```python
from build123d import *

# Parameters (mm, degrees)
F0_R     = 44.45
F1_DEPTH = 6.35


with BuildPart() as f1:
    # F0 (on Top) → F1 (new body)
    with BuildSketch(Plane.XY):
        Circle(F0_R)
        with BuildLine():
            ThreePointArc((26.940768, -26.940768), (0, -38.1), (-26.940768, -26.940768))
            ThreePointArc((-26.940768, -26.940768), (-35.19981, 14.580239), (0, 38.1))
            ThreePointArc((0, 38.1), (26.940768, 26.940768), (38.1, 0))
            ThreePointArc((38.1, 0), (35.19981, -14.580239), (26.940768, -26.940768))
        make_face(mode=Mode.SUBTRACT)
    extrude(amount=F1_DEPTH)


solid = f1.part
```
Geometry check sheet. Reference: the model listing, model coordinates, mm. Give positions to 0.01 mm unless a question says otherwise; leave off trailing zeros. Write each loop counter-clockwise with the first axis right and the second up, starting at its lowest first coordinate (ties: lowest second). Pieces come first, ordered by that corner, then holes. Notation, with made-up numbers: (65, 17) -> (71, 17) arc R13 cw to (71, 33) -> close; hole circle Ø7 at (-20.5, 48.25). An arc over 180 degrees is marked (long way). Use one line per item in the form item = value.
Item 1: Scan lines: line 1 (Y direction, x = -1, z = 6.25); line 2 (Y direction, x = 17.5, z = 1); line 3 (X direction, y = 24, z = 5.25). Record each from-to range of solid material in increasing order.
Results list:
line_1 = -44.44 to -38.09, 38.09 to 44.44
line_2 = -40.86 to -33.84, 33.84 to 40.86
line_3 = -37.41 to -29.59, 29.59 to 37.41
Item 2: Mould release check, pull along X, two halves, no side actions. Record for faces 1 (the cylindrical face through (42.397, 13.352, 3.131)), 2 (the flat face through (33, 20, 6.35)): released by +X, released by -X, zero draft, split by the parting line, or undercut.
Results list:
face_1 = split by the parting line
face_2 = zero draft
Item 3: Sectioned sample at C-C on y = -36.5. Enter the section's corners in (x, z).
Results list:
outline = (-25.37, 0) -> (-10.93, 0) -> (-10.93, 6.35) -> (-25.37, 6.35) -> close; (10.93, 0) -> (25.37, 0) -> (25.37, 6.35) -> (10.93, 6.35) -> close
Item 4: Sectioned sample at B-B on x = 15. Enter the section's corners in (y, z).
Results list:
outline = (-41.84, 0) -> (-35.02, 0) -> (-35.02, 6.35) -> (-41.84, 6.35) -> close; (35.02, 0) -> (41.84, 0) -> (41.84, 6.35) -> (35.02, 6.35) -> close
Item 5: Depth check by flat-ended pin: pin 1 Ø1 at (x, z) = (24.5, 4.5) entering from +Y. Enter the tip coordinate at first touch or a pass-through.
Results list:
pin_1 = 37.41
Item 6: Sectioned sample at A-A on z = 4.25. Enter the section's corners in (x, y).
Results list:
outline = circle Ø88.9 at (0, 0); hole (-26.94, -26.94) arc R38.1 ccw to (26.94, -26.94) arc R38.1 ccw to (38.1, 0) arc R38.1 ccw to (0, 38.1) arc R38.1 ccw to start
